```python
from build123d import *

# Parameters (mm, degrees)
SKETCH_1_W      = 60
SKETCH_1_H      = 11
SKETCH_1_R      = 1.55
EXTRUDE_1_DEPTH = 3
CHAMFER_1_SIZE  = 1.6


with BuildPart() as part:
    # 草图1 → 凸台-拉伸1 (new body)
    with BuildSketch(Plane.XY):
        Rectangle(SKETCH_1_W, SKETCH_1_H)
        with Locations((18, 2.5)):
            Circle(SKETCH_1_R, mode=Mode.SUBTRACT)
        with Locations((-2, 2.5)):
            Circle(SKETCH_1_R, mode=Mode.SUBTRACT)
        with Locations((0, -2.5)):
            Circle(SKETCH_1_R, mode=Mode.SUBTRACT)
        with Locations((18, -2.5)):
            Circle(SKETCH_1_R, mode=Mode.SUBTRACT)
        with Locations((-18, -2.5)):
            Circle(SKETCH_1_R, mode=Mode.SUBTRACT)
    extrude(amount=EXTRUDE_1_DEPTH)

    # 倒角1
    # the kernel refuses this chamfer: 1.6 mm, written as the material it takes off along each edge
    with BuildSketch(Plane(origin=(18, 2.5, 3), x_dir=(1, 0, 0), z_dir=(0, -1, 0))) as chamfer_1_piece_1:
        Polygon((1.55, -CHAMFER_1_SIZE), (1.55 + CHAMFER_1_SIZE, 0), (1.55, 0), align=None)
    revolve(axis=Axis((18, 2.5, 3), (0, 0, 1)), mode=Mode.SUBTRACT)
    with BuildSketch(Plane(origin=(-2, 2.5, 3), x_dir=(1, 0, 0), z_dir=(0, -1, 0))) as chamfer_1_piece_2:
        Polygon((1.55, -CHAMFER_1_SIZE), (1.55 + CHAMFER_1_SIZE, 0), (1.55, 0), align=None)
    revolve(axis=Axis((-2, 2.5, 3), (0, 0, 1)), mode=Mode.SUBTRACT)


solid = part.part
```
Part model, mm, in its own coordinate system. Give positions to 0.01 mm unless a question says otherwise; leave off trailing zeros. Order: outer loops, then holes, each group sorted by start corner. A loop starts at its lowest first (then second) coordinate and runs counter-clockwise, first axis right, second up. Notation, with made-up numbers: (79, 35.25) - (135, 35.25) arc R15 cw to (135, 59.25) - close; hole circle Ø4 at (76.5, -16.5). An arc over 180 degrees is marked (long way). Use one line per item in the form item = value.
Item 1: Probe probe 1 along Y at (x, z) = (18, 1); probe 2 along Y at (x, z) = (0, 1.8); probe 3 along X at (y, z) = (3.5, 0.65). List the from-to ranges inside material, lowest first. Write a range as from..to.
Solution:
probe_1 = -5.5..-4.05, -0.95..0.95, 4.05..5.5
probe_2 = -5.5..-4.05, -0.95..5.5
probe_3 = -30..-3.18, -0.82..16.82, 19.18..30
Item 2: Slice it at A-A on y = -2.5. Give the cut face in (x, z).
Solution:
outline = (-30, 0) - (-19.55, 0) - (-19.55, 3) - (-30, 3) - close; (-16.45, 0) - (-1.55, 0) - (-1.55, 3) - (-16.45, 3) - close; (1.55, 0) - (16.45, 0) - (16.45, 3) - (1.55, 3) - close; (19.55, 0) - (30, 0) - (30, 3) - (19.55, 3) - close
Item 3: Slice it at D-D on x = -18. Give the cut face in (y, z), and give its area (3 significant figures).
Solution:
outline = (-5.5, 0) - (-4.05, 0) - (-4.05, 3) - (-5.5, 3) - close; (-0.95, 0) - (5.5, 0) - (5.5, 3) - (-0.95, 3) - close
area = 23.7 mm2
Item 4: Slice it at C-C on x = 18. Give the cut face in (y, z).
Solution:
outline = (-5.5, 0) - (-4.05, 0) - (-4.05, 3) - (-5.5, 3) - close; (-0.95, 0) - (0.95, 0) - (0.95, 1.4) - (-0.65, 3) - (-0.95, 3) - close; (4.05, 0) - (5.5, 0) - (5.5, 2.85) - (4.05, 1.4) - close
Item 5: Slice it at B-B on z = 2.35. Give the cut face in (x, y), and give its area (3 significant figures).
Solution:
outline = (-30, -5.5) - (30, -5.5) - (30, 5.5) - (-30, 5.5) - close; hole circle Ø3.1 at (-18, -2.5); hole circle Ø5 at (-2, 2.5); hole circle Ø3.1 at (0, -2.5); hole circle Ø5 at (18, 2.5); hole circle Ø3.1 at (18, -2.5)
area = 598 mm2
Item 6: Two-plate mould, pull along Y, no slides. Class faces 1 (the face through (-30, 0, 1)), 2 (the face through (0, -5.5, 1)), 3 (the face through (-16.568, -3.094, 1.479)): released by +Y, released by -Y, zero draft, split by the parting line, or undercut.
Solution:
face_1 = zero draft
face_2 = released by -Y
face_3 = undercut
